The listing builds one solid part. Answer for the finished solid, in the listing's coordinates (mm). Face numbers are marked on the shaded views. A direction names the side the tool comes from. Round coordinates to 2 decimals unless told otherwise and drop trailing zeros. Order: outer loops, then holes, each group sorted by start corner. A loop starts at its lowest first (then second) coordinate and runs counter-clockwise, first axis right, second up. Notation, with made-up numbers: M -1,-2 L 53,-2 A21 cw 53,29 Z; hole C 88,67.5 d11. An arc over 180 degrees is marked long. Put each result on its own line as item: value. Start each with the question number.
1. The part is cut by section B-B (z = 33). Give the vertices of the cut face in (x, y).
2. The part is cut by section A-A (y = -17.5). Give the vertices of the cut face in (x, z).
3. Which of the six approach directions +Z, -Z, +X, -X, +Y, -Y give full straight-line access (tool end or side, diameter ignored) to the marked faces 5 and 6?
4. The mould has two halves that part along X. Classify the marked faces 1, 2, 3 and 4: +X half, -X half, draft (parallel to the pull), parting line (faces both ways), or undercut.
5. The part is cut by section C-C (x = 6.5). Give the vertices of the cut face in (y, z), then the cut area to 3 significant figures.
6. Each of these flat-tipped pins is pushed along its axis until it touches: pin 1 Ø1.2 at (x, y) = (1.5, -0.5) entering from +Z; pin 2 Ø6 at (x, z) = (4, -7) entering from -Y; pin 3 Ø0.6 at (x, z) = (10.5, -55) entering from +Y. Where does it stop, or does it pass through?
7. Consider line 1 (X direction, y = -10.5, z = 0.5); line 2 (Y direction, x = 1.75, z = -22.5); line 3 (Y direction, x = 9.75, z = -12). Determine where each line is inside the solid, lowest interval first.
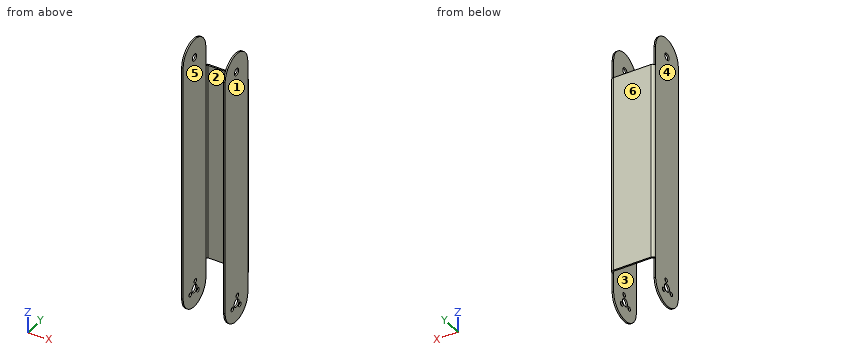
from build123d import *

# Parameters (mm, degrees)
SKETCH1_W                    = 18
SKETCH1_H                    = 100
BASE_FLANGE1_DEPTH           = 0.7366
EDGE_FLANGE1_DEPTH           = 100
EDGE_FLANGE1_BEND_DEPTH      = 100
SKETCH12_R                   = 2
TAB1_DEPTH                   = 0.7366
SKETCH15_R                   = 1.75
TAB2_DEPTH                   = 0.7366
F_2_05_2_05_DIAMETER_HOLE1_D = 2.05


# Sheet-metal steps are written as plain solids
with BuildPart() as part:
    # Sketch1 → Base-Flange1 (new body)
    with BuildSketch(Plane(origin=(0, 0, 0), x_dir=(1, 0, 0), z_dir=(0, 1, 0))):
        Rectangle(SKETCH1_W, SKETCH1_H)
    extrude(amount=-BASE_FLANGE1_DEPTH)

    # Edge-Flange1 section (across the edge) → Edge-Flange1 (add)
    with BuildSketch(Plane(origin=(10, -0.7366, -50), x_dir=(-1, 0, 0), z_dir=(0, 0, 1))):
        with BuildLine():
            Line((-0.7366, 0.7366), (-0.7366, 19.2634))
            Line((-0.7366, 19.2634), (0, 19.2634))
            Line((0, 19.2634), (0, 0.7366))
            ThreePointArc((0, 0.7366), (0.215745145, 0.215745145), (0.7366, 0))
            Line((0.7366, 0), (1, 0))
            Line((1, 0), (1, -0.7366))
            Line((1, -0.7366), (0.7366, -0.7366))
            ThreePointArc((0.7366, -0.7366), (-0.30510971, -0.30510971), (-0.7366, 0.7366))
        make_face()
    extrude(amount=EDGE_FLANGE1_DEPTH)

    # Edge-Flange1 section 2 (across the edge) → Edge-Flange1 bend (add)
    with BuildSketch(Plane(origin=(-10, -0.7366, 50), x_dir=(1, 0, 0), z_dir=(0, 0, -1))):
        with BuildLine():
            Line((-0.7366, 0.7366), (-0.7366, 19.2634))
            Line((-0.7366, 19.2634), (0, 19.2634))
            Line((0, 19.2634), (0, 0.7366))
            ThreePointArc((0, 0.7366), (0.215745145, 0.215745145), (0.7366, 0))
            Line((0.7366, 0), (1, 0))
            Line((1, 0), (1, -0.7366))
            Line((1, -0.7366), (0.7366, -0.7366))
            ThreePointArc((0.7366, -0.7366), (-0.30510971, -0.30510971), (-0.7366, 0.7366))
        make_face()
    extrude(amount=EDGE_FLANGE1_BEND_DEPTH)

    # Sketch12 → Tab1 (add)
    with BuildSketch(Plane.ZY.offset(10.7366)):
        with BuildLine():
            Line((-50, -1.4732), (-50, -20))
            Line((-50, -20), (-60, -20))
            ThreePointArc((-60, -20), (-69.2634, -10.7366), (-60, -1.4732))
            Line((-60, -1.4732), (-50, -1.4732))
        make_face()
        with Locations(Location((-60, -10.7366, 0), (0, 0, 270))):
            Circle(SKETCH12_R, mode=Mode.SUBTRACT)
    tab1 = extrude(amount=-TAB1_DEPTH)

    # Mirror1: Tab1 across plane
    add(tab1.mirror(Plane(origin=(0, 0, 0), x_dir=(0, 0, 1), z_dir=(1, 0, 0))))

    # Sketch15 → Tab2 (add)
    with BuildSketch(Plane(origin=(10.7366, 0, 0), x_dir=(0, 0, -1), z_dir=(1, 0, 0))):
        with BuildLine():
            Line((-50, -20), (-50, -1.4732))
            Line((-50, -1.4732), (-60, -1.4732))
            ThreePointArc((-60, -1.4732), (-69.2634, -10.7366), (-60, -20))
            Line((-60, -20), (-50, -20))
        make_face()
        with Locations(Location((-60, -10.7366, 0), (0, 0, 90))):
            Circle(SKETCH15_R, mode=Mode.SUBTRACT)
    tab2 = extrude(amount=-TAB2_DEPTH)

    # Mirror4: Tab2 across plane
    add(tab2.mirror(Plane(origin=(0, 0, 0), x_dir=(0, 0, 1), z_dir=(1, 0, 0))))

    # Ø2.05 (2.05) Diameter Hole1 (through all)
    with Locations(Plane(origin=(10.7366, -177.313180916, -73.74616676), x_dir=(0, 0.24782925197186137, -0.9688037272157182), z_dir=(1, 0, 0))):
        with Locations((24.667042937, 166.329840483), (30.950682453, 166.871449852), (28.277910167, 161.158853719)):
            Hole(F_2_05_2_05_DIAMETER_HOLE1_D / 2)


solid = part.part
Resolved:
1. outline: M -10.74,-20 L -10,-20 L -10,-1.47 A0.74 cw -9.26,-0.74 L 9.26,-0.74 A0.74 cw 10,-1.47 L 10,-20 L 10.74,-20 L 10.74,-1.47 A1.47 ccw 9.26,0 L -9.26,0 A1.47 ccw -10.74,-1.47 Z
2. outline: M -10.74,-66.33 L -10,-66.33 L -10,66.33 L -10.74,66.33 Z; M 10,-66.33 L 10.74,-66.33 L 10.74,66.33 L 10,66.33 Z
3. face 5: +Z, -Z, -Y
3. face 6: +Z, -Z, +X, -X, +Y
4. face 1: +X half
4. face 2: undercut
4. face 3: undercut
4. face 4: -X half
5. outline: M -0.74,-50 L 0,-50 L 0,50 L -0.74,50 Z
5. area: 73.7 mm2
6. pin 1: z = 50
6. pin 2: y = -0.74
6. pin 3: y = -1.47
7. line 1: -10.74 to -10, 10 to 10.74
7. line 2: -0.74 to 0
7. line 3: -0.92 to -0.08
